The figure shows three views and two pictorial views of one solid part (mm, origin at its lowest corner). Answer the questions. Give positions to 0.01 mm unless a question says otherwise; leave off trailing zeros. Order: outer loops, then holes, each group sorted by start corner. A loop starts at its lowest first (then second) coordinate and runs counter-clockwise, first axis right, second up. Notation, with made-up numbers: M -36,-20.75 L 13,-20.75 A16 cw 13,8.25 Z; hole C 38,-2 d3. An arc over 180 degrees is marked long. One line per item, written item: value. Start each with the question number.
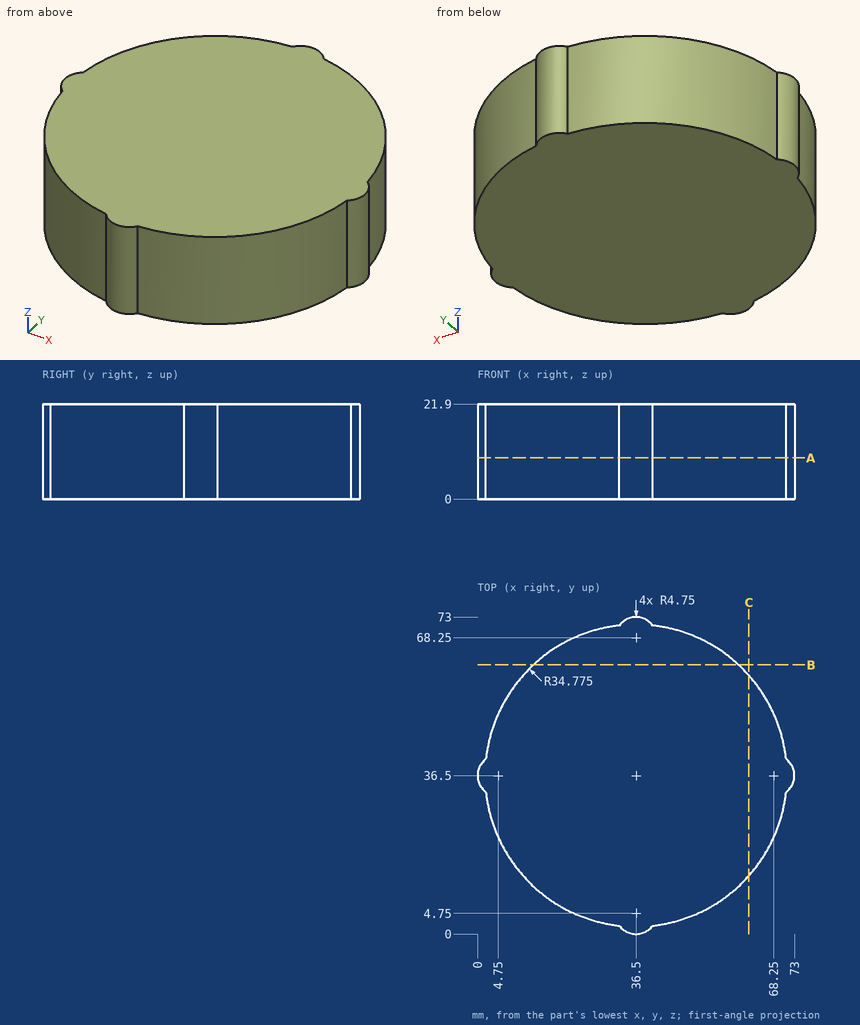
Q1. Each of these flat-tipped pins is pushed along its axis until it touches: pin 1 (10 mm diameter, centred on y = 62, z = 7, fed in from -X); pin 2 (5 mm diameter, centred on y = 14.5, z = 9, fed in from +X); pin 3 (12 mm diameter, centred on x = 51, z = 7, fed in from -Y); pin 4 (1.5 mm diameter, centred on x = 27.5, y = 34, fed in from -Z). Where does it stop, or does it pass through?
Q2. Find section B-B, the plane y = 62. Give the vertices of the cut face in (x, z).
Q3. Consider probe 1 along X at (y, z) = (38.5, 8.25); probe 2 along Y at (x, z) = (41, 13.75). Determine where each line is inside the solid, lowest interval first.
Q4. Find section C-C, the plane x = 62.5. Give the vertices of the cut face in (y, z), then the cut area to 3 significant figures.
Q5. Find section A-A, the plane z = 9.5. Give the vertices of the cut face in (x, y) (3 decimals).
Evaluation:
1. pin 1: x = 8.41
1. pin 2: x = 65.29
1. pin 3: y = 2.78
1. pin 4: z = 0
2. outline: M 12.86,0 L 60.14,0 L 60.14,21.9 L 12.86,21.9 Z
3. probe 1: 0.44 to 72.56
3. probe 2: 2.02 to 70.98
4. outline: M 13.41,0 L 59.59,0 L 59.59,21.9 L 13.41,21.9 Z
4. area: 1,010 mm2
5. outline: M 1.936,32.673 A34.775 ccw 32.673,1.936 A4.75 ccw 40.327,1.936 A34.775 ccw 71.064,32.673 A4.75 ccw 71.064,40.327 A34.775 ccw 40.327,71.064 A4.75 ccw 32.673,71.064 A34.775 ccw 1.936,40.327 A4.75 ccw Z
